Design review of the part built by this model. Coordinates are the model's own, in mm. A direction names the side the tool comes from. Give positions to 0.01 mm unless a question says otherwise; leave off trailing zeros. Write each loop counter-clockwise with the first axis right and the second up, starting at its lowest first coordinate (ties: lowest second). Pieces come first, ordered by that corner, then holes. Notation, with made-up numbers: (68, 2.5) -> (95, 2.5) arc R26 ccw to (95, 38.5) -> close; hole circle Ø5 at (64.5, 50). An arc over 180 degrees is marked (long way). Use CSV: the item, a comma, the result in double quotes.
```python
from build123d import *

# Parameters (mm, degrees)
SKETCH2_R           = 32.004
SKETCH2_R_2         = 14.326331359
SKETCH2_R_3         = 3.96875
BOSS_EXTRUDE3_DEPTH = 4.7625
FILLET2_R           = 2.54
FILLET3_R           = 2.54
FILLET4_R           = 2.54
FILLET5_R           = 2.54
SKETCH3_W           = 27.93619
SKETCH3_H           = 27.930200018
CUT_EXTRUDE1_DEPTH  = 4.7625
FILLET6_R           = 2.54
FILLET7_R           = 2.54


with BuildPart() as part:
    # Sketch2 → Boss-Extrude3 (new body)
    with BuildSketch(Plane.XY):
        with BuildLine():
            Line((-161.665509466, 75.768206346), (-31.830687389, 75.768206346))
            ThreePointArc((-31.830687389, 75.768206346), (-21.757108739, 67.512054819), (-14.51238939, 56.688235417))
            Line((-14.51238939, 56.688235417), (-14.51238939, -121.111764583))
            Line((-14.51238939, -121.111764583), (-178.60400939, -121.111764583))
            Line((-178.60400939, -121.111764583), (-178.60400939, 56.688235417))
            ThreePointArc((-178.60400939, 56.688235417), (-171.519463205, 67.457510218), (-161.665509466, 75.768206346))
        make_face()
        with Locations(Location((-137.96400939, 37.668206346, 0), (0, 0, 180))):
            Circle(SKETCH2_R, mode=Mode.SUBTRACT)
        with Locations(Location((-55.15238939, 37.668206346, 0), (0, 0, 180))):
            Circle(SKETCH2_R, mode=Mode.SUBTRACT)
        with Locations(Location((-96.30038939, -8.051793654, 0), (0, 0, 180))):
            Circle(SKETCH2_R_2, mode=Mode.SUBTRACT)
        with Locations(Location((-35.74551939, -8.051793654, 0), (0, 0, 180))):
            Circle(SKETCH2_R_3, mode=Mode.SUBTRACT)
        with Locations(Location((-156.85525939, -8.051793654, 0), (0, 0, 180))):
            Circle(SKETCH2_R_3, mode=Mode.SUBTRACT)
        with Locations(Location((-168.077299629, -106.909902872, 0), (0, 0, 180))):
            Circle(SKETCH2_R_3, mode=Mode.SUBTRACT)
        with Locations(Location((-96.30038939, -107.174765002, 0), (0, 0, 180))):
            Circle(SKETCH2_R_3, mode=Mode.SUBTRACT)
        Polygon((-119.16038939, -45.520207297), (-119.16038939, -76.631793654), (-119.16038939, -107.199674954), (-159.049264091, -106.297978958), (-119.16038939, -9.66645302), align=None, mode=Mode.SUBTRACT)
        Polygon((-73.44038939, -45.520207297), (-73.44038939, -76.631793654), (-73.44038939, -107.174765002), (-50.06857939, -107.174765002), (-50.06857939, -85.561564565), (-42.111373674, -85.561564565), (-73.44038939, -9.66645302), align=None, mode=Mode.SUBTRACT)
        with BuildLine():
            Line((-165.90400939, -8.051793654), (-165.90400939, -72.234249773))
            Line((-165.90400939, -72.234249773), (-165.90400939, -98.126015002))
            Line((-165.90400939, -98.126015002), (-127.899360964, -6.059061553))
            ThreePointArc((-127.899360964, -6.059061553), (-137.96400939, -7.202397682), (-148.028657817, -6.059061553))
            ThreePointArc((-148.028657817, -6.059061553), (-155.852721218, -17.044835062), (-165.90400939, -8.051793654))
        make_face(mode=Mode.SUBTRACT)
        with BuildLine():
            Line((-26.69676939, -8.051793654), (-26.69676939, -72.234249773))
            Line((-26.69676939, -72.234249773), (-26.69676939, -85.561564565))
            Line((-26.69676939, -85.561564565), (-31.883294019, -85.561564565))
            Line((-31.883294019, -85.561564565), (-64.701417817, -6.059061553))
            ThreePointArc((-64.701417817, -6.059061553), (-54.63676939, -7.202397682), (-44.572120964, -6.059061553))
            ThreePointArc((-44.572120964, -6.059061553), (-36.748057563, -17.044835062), (-26.69676939, -8.051793654))
        make_face(mode=Mode.SUBTRACT)
        with BuildLine():
            Line((-110.27038939, -107.174765002), (-105.34913939, -107.174765002))
            ThreePointArc((-105.34913939, -107.174765002), (-96.30038939, -98.126015002), (-87.25163939, -107.174765002))
            Line((-87.25163939, -107.174765002), (-82.33038939, -107.174765002))
            Line((-82.33038939, -107.174765002), (-82.33038939, -69.074765002))
            Line((-82.33038939, -69.074765002), (-110.27038939, -69.074765002))
            Line((-110.27038939, -69.074765002), (-110.27038939, -107.174765002))
        make_face(mode=Mode.SUBTRACT)
        with BuildLine():
            Line((-105.751769429, 69.672206346), (-85.417792119, 69.672206346))
            ThreePointArc((-85.417792119, 69.672206346), (-91.388421836, 62.588949087), (-95.759407575, 54.420997306))
            ThreePointArc((-95.759407575, 54.420997306), (-99.982218631, 62.553302087), (-105.751769429, 69.672206346))
        make_face(mode=Mode.SUBTRACT)
        with BuildLine():
            Line((-110.27038939, -30.911793654), (-110.27038939, -61.454765002))
            Line((-110.27038939, -61.454765002), (-82.33038939, -61.454765002))
            Line((-82.33038939, -61.454765002), (-82.33038939, -30.911793654))
            ThreePointArc((-82.33038939, -30.911793654), (-96.30038939, -34.842473003), (-110.27038939, -30.911793654))
        make_face(mode=Mode.SUBTRACT)
    extrude(amount=BOSS_EXTRUDE3_DEPTH)

    # Fillet2
    fillet2_edges = [part.edges().sort_by_distance(p)[0] for p in [
        (-82.33038939, -30.911793654, 2.38125),
        (-110.27038939, -30.911793654, 2.38125),
        (-148.028657817, -6.059061553, 2.38125),
        (-165.90400939, -8.051793654, 2.38125),
        (-26.69676939, -8.051793654, 2.38125),
        (-44.572120964, -6.059061553, 2.38125),
    ]]
    fillet(fillet2_edges, radius=FILLET2_R)

    # Fillet3
    fillet3_edges = [part.edges().sort_by_distance(p)[0] for p in [
        (-110.27038939, -61.454765002, 2.38125),
        (-82.33038939, -61.454765002, 2.38125),
        (-110.27038939, -107.174765002, 2.38125),
        (-105.34913939, -107.174765002, 2.38125),
        (-87.25163939, -107.174765002, 2.38125),
        (-82.33038939, -107.174765002, 2.38125),
        (-73.44038939, -107.174765002, 2.38125),
        (-50.06857939, -107.174765002, 2.38125),
        (-119.16038939, -107.199674954, 2.38125),
        (-26.69676939, -85.561564565, 2.38125),
    ]]
    fillet(fillet3_edges, radius=FILLET3_R)

    # Fillet4
    fillet4_edges = [part.edges().sort_by_distance(p)[0] for p in [
        (-82.33038939, -69.074765002, 2.38125),
        (-110.27038939, -69.074765002, 2.38125),
    ]]
    fillet(fillet4_edges, radius=FILLET4_R)

    # Fillet5
    fillet5_edges = [part.edges().sort_by_distance(p)[0] for p in [
        (-95.759407575, 54.420997306, 2.38125),
        (-85.417792119, 69.672206346, 2.38125),
        (-105.751769429, 69.672206346, 2.38125),
    ]]
    fillet(fillet5_edges, radius=FILLET5_R)

    # Sketch3 → Cut-Extrude1 (cut)
    with BuildSketch(Plane.XY.offset(4.7625)):
        with Locations((-28.48048439, -107.146664574)):
            Rectangle(SKETCH3_W, SKETCH3_H)
    extrude(amount=-CUT_EXTRUDE1_DEPTH, mode=Mode.SUBTRACT)

    # Fillet6
    fillet6_edges = [part.edges().sort_by_distance(p)[0] for p in [
        (-14.51238939, 56.688235417, 2.38125),
        (-178.60400939, -121.111764583, 2.38125),
        (-178.60400939, 56.688235417, 2.38125),
        (-161.665509466, 75.768206346, 2.38125),
        (-31.830687389, 75.768206346, 2.38125),
        (-14.51238939, -93.181564565, 2.38125),
        (-42.44857939, -121.111764583, 2.38125),
        (-42.44857939, -93.181564565, 2.38125),
    ]]
    fillet(fillet6_edges, radius=FILLET6_R)

    # Fillet7
    fillet7_edges = [part.edges().sort_by_distance(p)[0] for p in [
        (-73.44038939, -9.66645302, 2.38125),
        (-50.06857939, -85.561564565, 2.38125),
        (-42.111373674, -85.561564565, 2.38125),
        (-119.16038939, -9.66645302, 2.38125),
        (-159.049264091, -106.297978958, 2.38125),
        (-165.90400939, -98.126015002, 2.38125),
        (-127.899360964, -6.059061553, 2.38125),
        (-64.701417817, -6.059061553, 2.38125),
        (-31.883294019, -85.561564565, 2.38125),
    ]]
    fillet(fillet7_edges, radius=FILLET7_R)


solid = part.part
```
(1) Take a section at A-A (y = 20.5). Write out the cut boundary in (x, z).
Established:
outline,"(-178.6, 0) -> (-164.97, 0) -> (-164.97, 4.76) -> (-178.6, 4.76) -> close; (-110.95, 0) -> (-82.16, 0) -> (-82.16, 4.76) -> (-110.95, 4.76) -> close; (-28.14, 0) -> (-14.51, 0) -> (-14.51, 4.76) -> (-28.14, 4.76) -> close"
(2) For line 1 along Y through (x, z) = (-65, 0.65); line 2 along X through (y, z) = (20.5, 3.6); line 3 along X through (y, z) = (24.5, 3.9), list the stretches that pass through material, from the lowest coordinate up. Write a range as [from, to].
Established:
line 1,"y = [-121.11, -107.17], [-30.11, 7.22], [68.12, 75.77]"
line 2,"x = [-178.6, -164.97], [-110.95, -82.16], [-28.14, -14.51]"
line 3,"x = [-178.6, -167.13], [-108.79, -84.32], [-25.98, -14.51]"
(3) Clearance check with flat-ended pins moving along their axes: pin 1 (8 mm diameter, centred on x = -73, y = -44, fed in from +Z); pin 2 (2.5 mm diameter, centred on y = -112, z = 3, fed in from +X). State where each tip first meets the part, or that it passes through.
Established:
pin 1,"stops at z = 4.76"
pin 2,"stops at x = -42.45"
(4) Take a section at B-B (x = -79.5). Write out the cut boundary in (y, z), then the cut area to 3 significant figures.
Established:
outline,"(-121.11, 0) -> (16.9, 0) -> (16.9, 4.76) -> (-121.11, 4.76) -> close; (58.44, 0) -> (75.77, 0) -> (75.77, 4.76) -> (58.44, 4.76) -> close"
area,"740 mm2"
(5) Tool access review of faces 4 (the face through (-91.46, 62.48, 2.35)), 5 (the face through (-178.604, -32, 2)): name each direction out of +Z, -Z, +X, -X, +Y, -Y from which nothing blocks a thin tool from reaching the whole face with its end or side.
Established:
face 4,"+Z, -Z"
face 5,"+Z, -Z, -X, +Y, -Y"
(6) Mouldability with a two-part tool opening along X and no side actions: class faces 1 (the face through (-77, -21, 4.762)), 2 (the face through (-119.16, -63, 2)), 3 (the face through (-171.689, 67.266, 2.348)) as +X half, -X half, draft (parallel to the pull), parting line (faces both ways), or undercut.
Established:
face 1,"draft"
face 2,"undercut"
face 3,"-X half"
(7) Take a section at C-C (y = -1.5). Write out the cut boundary in (x, z), then the cut area to 3 significant figures.
Established:
outline,"(-178.6, 0) -> (-109.04, 0) -> (-109.04, 4.76) -> (-178.6, 4.76) -> close; (-83.56, 0) -> (-14.51, 0) -> (-14.51, 4.76) -> (-83.56, 4.76) -> close"
area,"660 mm2"
(8) Take a section at D-D (y = -77). Write out the cut boundary in (x, z), then the cut area to 3 significant figures.
Established:
outline,"(-178.6, 0) -> (-165.9, 0) -> (-165.9, 4.76) -> (-178.6, 4.76) -> close; (-157.18, 0) -> (-146.96, 0) -> (-146.96, 4.76) -> (-157.18, 4.76) -> close; (-119.16, 0) -> (-110.27, 0) -> (-110.27, 4.76) -> (-119.16, 4.76) -> close; (-82.33, 0) -> (-73.44, 0) -> (-73.44, 4.76) -> (-82.33, 4.76) -> close; (-45.65, 0) -> (-35.42, 0) -> (-35.42, 4.76) -> (-45.65, 4.76) -> close; (-26.7, 0) -> (-14.51, 0) -> (-14.51, 4.76) -> (-26.7, 4.76) -> close"
area,"301 mm2"
